Geometry: final body of the model. Coordinates: model frame, mm. Round coordinates to 2 decimals unless told otherwise and drop trailing zeros. Write each loop counter-clockwise with the first axis right and the second up, starting at its lowest first coordinate (ties: lowest second). Pieces come first, ordered by that corner, then holes. Notation, with made-up numbers: (75.5, -33) - (89.5, -33) arc R8 ccw to (89.5, -23) - close; hole circle Ø1 at (51.25, 52.5). An arc over 180 degrees is marked (long way). Write each question's results on one line, items separated by ' | '.
from build123d import *

# Parameters (mm, degrees)
F1_DEPTH = 6
F2_DEPTH = 15
F5_D     = 10.5
F5_DEPTH = 8
F5_TIP   = 3.1545182499
F6_D     = 9
F6_DEPTH = 8
F6_TIP   = 2.7038727856


with BuildPart() as f1:
    # F0 (on Top) → F1 (new body)
    with BuildSketch(Plane.XY):
        with BuildLine():
            ThreePointArc((0, 9), (6.3639610307, 6.3639610307), (9, 0))
            Line((9, 0), (10, 0))
            ThreePointArc((10, 0), (9.9114443967, 1.327881761), (9.6473460058, 2.6322452478))
            Line((9.6473460058, 2.6322452478), (5.8095664532, 17.4996458335))
            ThreePointArc((5.8095664532, 17.4996458335), (3.6743791992, 20.7433044917), (0, 22))
            Line((0, 22), (0, 19.3))
            ThreePointArc((0, 19.3), (2.3334523779, 18.3334523779), (3.3, 16))
            ThreePointArc((3.3, 16), (2.3334523779, 13.6665476221), (0, 12.7))
            Line((0, 12.7), (0, 9))
        make_face()
        with BuildLine():
            ThreePointArc((-9, 0), (-6.3639610307, 6.3639610307), (0, 9))
            Line((0, 9), (0, 12.7))
            ThreePointArc((0, 12.7), (-3.3, 16), (0, 19.3))
            Line((0, 19.3), (0, 22))
            ThreePointArc((0, 22), (-3.6743791992, 20.7433044917), (-5.8095664532, 17.4996458335))
            Line((-5.8095664532, 17.4996458335), (-9.6473460058, 2.6322452478))
            ThreePointArc((-9.6473460058, 2.6322452478), (-9.9114443967, 1.327881761), (-10, 0))
            Line((-10, 0), (-9, 0))
        make_face()
        with BuildLine():
            Line((0, -12.7), (0, -9))
            ThreePointArc((0, -9), (-6.3639610307, -6.3639610307), (-9, 0))
            Line((-9, 0), (-10, 0))
            ThreePointArc((-10, 0), (-9.9114443967, -1.327881761), (-9.6473460058, -2.6322452478))
            Line((-9.6473460058, -2.6322452478), (-5.8095664532, -17.4996458335))
            ThreePointArc((-5.8095664532, -17.4996458335), (-3.6743791992, -20.7433044917), (0, -22))
            Line((0, -22), (0, -19.3))
            ThreePointArc((0, -19.3), (-3.3, -16), (0, -12.7))
        make_face()
        with BuildLine():
            Line((10, 0), (9, 0))
            ThreePointArc((9, 0), (6.3639610307, -6.3639610307), (0, -9))
            Line((0, -9), (0, -12.7))
            ThreePointArc((0, -12.7), (2.3334523779, -13.6665476221), (3.3, -16))
            ThreePointArc((3.3, -16), (2.3334523779, -18.3334523779), (0, -19.3))
            Line((0, -19.3), (0, -22))
            ThreePointArc((0, -22), (3.6743791992, -20.7433044917), (5.8095664532, -17.4996458335))
            Line((5.8095664532, -17.4996458335), (9.6473460058, -2.6322452478))
            ThreePointArc((9.6473460058, -2.6322452478), (9.9114443967, -1.327881761), (10, 0))
        make_face()
    extrude(amount=F1_DEPTH)

    # F0 (on Top) → F2 (join)
    with BuildSketch(Plane.XY):
        with BuildLine():
            ThreePointArc((-9, 0), (-6.3639610307, -6.3639610307), (0, -9))
            Line((0, -9), (0, 0))
            Line((0, 0), (-9, 0))
        make_face()
        with BuildLine():
            Line((0, 0), (0, 9))
            ThreePointArc((0, 9), (-6.3639610307, 6.3639610307), (-9, 0))
            Line((-9, 0), (0, 0))
        make_face()
        with BuildLine():
            Line((0, 0), (9, 0))
            ThreePointArc((9, 0), (6.3639610307, 6.3639610307), (0, 9))
            Line((0, 9), (0, 0))
        make_face()
        with BuildLine():
            ThreePointArc((0, -9), (6.3639610307, -6.3639610307), (9, 0))
            Line((9, 0), (0, 0))
            Line((0, 0), (0, -9))
        make_face()
    extrude(amount=F2_DEPTH)

    # F5
    with Locations(Plane.XY.offset(15)):
        with Locations((0, 0)):
            Hole(F5_D / 2, depth=F5_DEPTH)
            with Locations((0, 0, -(F5_DEPTH + F5_TIP / 2))):  # 118° drill point
                Cone(0, F5_D / 2, F5_TIP, mode=Mode.SUBTRACT)

    # F6
    with Locations(Plane(origin=(0, 0, 0), x_dir=(1, 0, 0), z_dir=(0, 0, -1))):
        with Locations((0, 0)):
            Hole(F6_D / 2, depth=F6_DEPTH)
            with Locations((0, 0, -(F6_DEPTH + F6_TIP / 2))):  # 118° drill point
                Cone(0, F6_D / 2, F6_TIP, mode=Mode.SUBTRACT)


solid = f1.part
Q1. Pin query (flat end, axial travel): pin 1 (4 mm diameter, centred on x = -3, z = 12.5, fed in from -Y); pin 2 (1.5 mm diameter, centred on x = 6, y = 9.5, fed in from +Z); pin 3 (6 mm diameter, centred on x = 1.5, z = 11, fed in from +Y). Return the tip coordinate at first contact, or that it passes through.
Answer block:
pin 1: y = -8.94 | pin 2: z = 6 | pin 3: y = 9
Q2. Section query D-D, the plane y = -8. Return loops of the section in (x, z), plus the area to 3 significant figures.
Answer block:
outline: (-8.26, 0) - (8.26, 0) - (8.26, 6) - (4.12, 6) - (4.12, 15) - (-4.12, 15) - (-4.12, 6) - (-8.26, 6) - close | area: 173 mm2
Q3. Ray query, line 1 along X through (y, z) = (0, 12.5); line 2 along X through (y, z) = (1.5, 3.75). Return the intervals inside material, ascending.
Answer block:
line 1: -9 to -5.25, 5.25 to 9 | line 2: -9.89 to -4.24, 4.24 to 9.89
Q4. Section query B-B, the plane y = 15.5. Return loops of the section in (x, z), plus the area to 3 significant figures.
Answer block:
outline: (-6.33, 0) - (-3.26, 0) - (-3.26, 6) - (-6.33, 6) - close; (3.26, 0) - (6.33, 0) - (6.33, 6) - (3.26, 6) - close | area: 36.8 mm2
Q5. Section query C-C, the plane z = 13. Return loops of the section in (x, y).
Answer block:
outline: circle Ø18 at (0, 0); hole circle Ø10.5 at (0, 0)
Q6. Section query A-A, the plane z = 1.75. Return loops of the section in (x, y).
Answer block:
outline: (-9.65, -2.63) - (-5.81, -17.5) arc R6 ccw to (5.81, -17.5) - (9.65, -2.63) arc R10 ccw to (9.65, 2.63) - (5.81, 17.5) arc R6 ccw to (-5.81, 17.5) - (-9.65, 2.63) arc R10 ccw to start; hole circle Ø9 at (0, 0); hole circle Ø6.6 at (0, -16); hole circle Ø6.6 at (0, 16)
Q7. Mould query, pull axis Y, two halves, no side actions, for faces 1 (the flat face through (7.7, -10.17, 2.96)), 2 (the flat face through (-0.1, -9.5, 6)), 3 (the cylindrical face through (-5, 1.6, 10.9)). Classes: pulls with the +Y half, pulls with the -Y half, needs draft (parallel to the pull), parting line crosses it, or undercut.
Answer block:
face 1: pulls with the -Y half | face 2: needs draft | face 3: undercut
